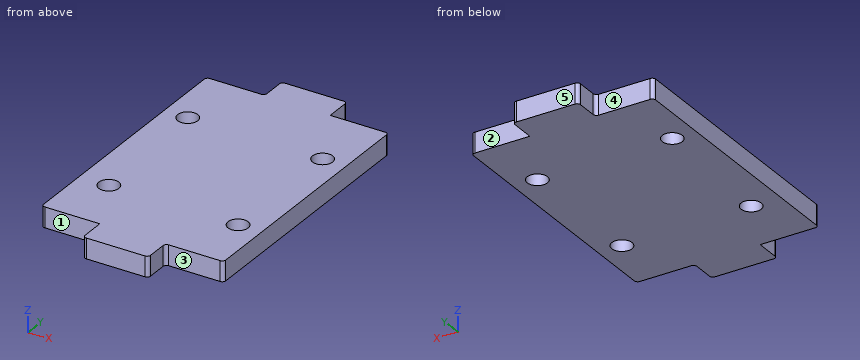
from build123d import *

# Parameters (mm, degrees)
ESQUISSE1_R        = 1.5
BOSS_EXTRU_1_DEPTH = 3
CONG_1_R           = 0.5


with BuildPart() as part:
    # Esquisse1 → Boss.-Extru.1 (new body)
    with BuildSketch(Plane.XY):
        Polygon((-13.5, 19.5), (-4.85133507, 19.5), (-4.85133507, 23.5), (4.85133507, 23.5), (4.85133507, 19.5), (13.5, 19.5), (13.5, -19.5), (4.85133507, -19.5), (4.85133507, -23.5), (-4.85133507, -23.5), (-4.85133507, -19.5), (-13.5, -19.5), align=None)
        with Locations((-10, 9.5)):
            Circle(ESQUISSE1_R, mode=Mode.SUBTRACT)
        with Locations(Location((10, 9.5, 0), (0, 0, 180))):
            Circle(ESQUISSE1_R, mode=Mode.SUBTRACT)
        with Locations((-9.158491979, -10.5)):
            Circle(ESQUISSE1_R, mode=Mode.SUBTRACT)
        with Locations(Location((10, -10.5, 0), (0, 0, 180))):
            Circle(ESQUISSE1_R, mode=Mode.SUBTRACT)
    extrude(amount=BOSS_EXTRU_1_DEPTH)

    # Congé1
    cong_1_edges = [part.edges().sort_by_distance(p)[0] for p in [
        (-13.5, 19.5, 1.5),
        (-4.85133507, 19.5, 1.5),
        (-4.85133507, 23.5, 1.5),
        (4.85133507, 23.5, 1.5),
        (13.5, 19.5, 1.5),
        (13.5, -19.5, 1.5),
        (4.85133507, -19.5, 1.5),
        (4.85133507, -23.5, 1.5),
        (-4.85133507, -23.5, 1.5),
        (-13.5, -19.5, 1.5),
    ]]
    fillet(cong_1_edges, radius=CONG_1_R)


solid = part.part
Geometry check sheet. Reference: the model listing, model coordinates, mm. Face numbers are marked on the shaded views. A direction names the side the tool comes from. Round coordinates to 2 decimals unless told otherwise and drop trailing zeros. Loops run counter-clockwise (first coordinate to the right, second up) from the corner with the lowest first, then second, coordinate; pieces in that order, holes last. Notation, with made-up numbers: (-3, 35) - (44, 35) arc R11 ccw to (44, 54) - close; hole circle Ø1 at (89.25, -18). An arc over 180 degrees is marked (long way). One line per question, with ' | ' between items. Start each with the question number.
1. Scan lines: line 1 (Y direction, x = 10, z = 2.05); line 2 (Y direction, x = -10, z = 1.9); line 3 (Y direction, x = -5.75, z = 2.05). Record each from-to range of solid material in increasing order. Write a range as [from, to].
2. Cross-section at A-A on y = 9.5. Record the cut outline in (x, z), then the cut area to 3 significant figures.
3. Depth check by flat-ended pin: pin 1 (1.5 mm diameter, centred on x = -10.5, z = 1, fed in from +Y); pin 2 (3.5 mm diameter, centred on x = 10, y = 9.5, fed in from -Z); pin 3 (0.9 mm diameter, centred on x = -8.5, z = 1, fed in from -Y); pin 4 (1.5 mm diameter, centred on y = -22, z = 2, fed in from -X). Enter the tip coordinate at first touch or a pass-through.
4. Cross-section at B-B on z = 0.5. Record the cut outline in (x, y).
5. Cross-section at C-C on x = -10. Record the cut outline in (y, z).
6. Cross-section at D-D on x = -6. Record the cut outline in (y, z).
7. Tool access check on the marked faces 1, 2, 3, 4 and 5. Record the directions out of +Z, -Z, +X, -X, +Y, -Y that give a thin tool (end or side, any length) a straight path to the whole face; none if there is none.
Taken from the geometry:
1) line 1: [-19.5, -12], [-9, 8], [11, 19.5] | line 2: [-19.5, -11.74], [-9.26, 8], [11, 19.5] | line 3: [-19.5, 19.5]
2) outline: (-13.5, 0) - (-11.5, 0) - (-11.5, 3) - (-13.5, 3) - close; (-8.5, 0) - (8.5, 0) - (8.5, 3) - (-8.5, 3) - close; (11.5, 0) - (13.5, 0) - (13.5, 3) - (11.5, 3) - close | area: 63.0 mm²
3) pin 1: y = 19.5 | pin 2: z = 0 | pin 3: y = -19.5 | pin 4: x = -4.85
4) outline: (-13.5, -19) arc R0.5 ccw to (-13, -19.5) - (-4.85, -19.5) - (-4.85, -23) arc R0.5 ccw to (-4.35, -23.5) - (4.35, -23.5) arc R0.5 ccw to (4.85, -23) - (4.85, -20) arc R0.5 cw to (5.35, -19.5) - (13, -19.5) arc R0.5 ccw to (13.5, -19) - (13.5, 19) arc R0.5 ccw to (13, 19.5) - (4.85, 19.5) - (4.85, 23) arc R0.5 ccw to (4.35, 23.5) - (-4.35, 23.5) arc R0.5 ccw to (-4.85, 23) - (-4.85, 20) arc R0.5 cw to (-5.35, 19.5) - (-13, 19.5) arc R0.5 ccw to (-13.5, 19) - close; hole circle Ø3 at (-10, 9.5); hole circle Ø3 at (-9.16, -10.5); hole circle Ø3 at (10, -10.5); hole circle Ø3 at (10, 9.5)
5) outline: (-19.5, 0) - (-11.74, 0) - (-11.74, 3) - (-19.5, 3) - close; (-9.26, 0) - (8, 0) - (8, 3) - (-9.26, 3) - close; (11, 0) - (19.5, 0) - (19.5, 3) - (11, 3) - close
6) outline: (-19.5, 0) - (19.5, 0) - (19.5, 3) - (-19.5, 3) - close
7) face 1: +Z, -Z, -X, -Y | face 2: +Z, -Z, +X, +Y | face 3: +Z, -Z, +X, -Y | face 4: +Z, -Z, -X, +Y | face 5: +Z, -Z, +X, -X, +Y
